Work out the finished part from the listing and answer in its coordinate system (mm). Round coordinates to 2 decimals unless told otherwise and drop trailing zeros. Loops run counter-clockwise (first coordinate to the right, second up) from the corner with the lowest first, then second, coordinate; pieces in that order, holes last. Notation, with made-up numbers: (-26, 33.25) -> (8, 33.25) arc R5 ccw to (8, 38.25) -> close; hole circle Ø4 at (-9.5, -2.75). An arc over 180 degrees is marked (long way). Write item = value, one per line. Start each with the question number.
```python
from build123d import *

# Parameters (mm, degrees)
BOSS_EXTRUDE1_DEPTH  = 3
M5_CLEARANCE_HOLE1_D = 5.5
M5_CLEARANCE_HOLE2_D = 5.5
M5_CLEARANCE_HOLE3_D = 5.5
FILLET2_R            = 2.5


with BuildPart() as part:
    # Sketch1 → Boss-Extrude1 (new body)
    with BuildSketch(Plane.XY):
        with BuildLine():
            Line((8.695255676, -3.826555727), (2.390511351, -18.153111454))
            ThreePointArc((2.390511351, -18.153111454), (-4.61754166, -26.412402673), (-15, -29.5))
            Line((-15, -29.5), (-51.88, -29.5))
            Line((-51.88, -29.5), (-51.88, -10.5))
            Line((-51.88, -10.5), (-15, -10.5))
            Line((-15, -10.5), (-8.695255676, 3.826555727))
            ThreePointArc((-8.695255676, 3.826555727), (3.826555727, 8.695255676), (8.695255676, -3.826555727))
        make_face()
    extrude(amount=BOSS_EXTRUDE1_DEPTH)

    # M5 Clearance Hole1 (through all)
    with Locations(Plane.XY.offset(3)):
        with Locations((-43.44, -20)):
            Hole(M5_CLEARANCE_HOLE1_D / 2)

    # M5 Clearance Hole2 (through all)
    with Locations(Plane.XY.offset(3)):
        with Locations((-23.44, -20)):
            Hole(M5_CLEARANCE_HOLE2_D / 2)

    # M5 Clearance Hole3 (through all)
    with Locations(Plane.XY.offset(3)):
        with Locations((0, 0)):
            Hole(M5_CLEARANCE_HOLE3_D / 2)

    # Fillet2
    fillet2_edges = [part.edges().sort_by_distance(p)[0] for p in [
        (-51.88, -29.5, 1.5),
        (-51.88, -10.5, 1.5),
        (-15, -10.5, 1.5),
    ]]
    fillet(fillet2_edges, radius=FILLET2_R)


solid = part.part
```
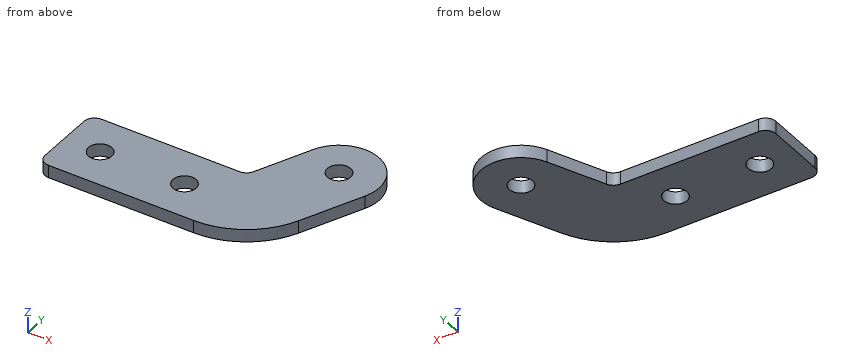
Item 1: Section A-A (x = -23.44) is taken. Determine the outline of the cut face in (y, z), then the cut area to 3 significant figures.
Item 2: Section B-B (z = 1.25) is taken. Determine the outline of the cut face in (x, y).
Item 3: Find the intervals of material crossed by line 1 along Y through (x, z) = (-23.44, 1.1); line 2 along X through (y, z) = (-17.5, 1.9); line 3 along X through (y, z) = (-22, 2.55), in increasing order. Write a range as [from, to].
Item 4: Flat-ended cylindrical pins translate along their axes: pin 1 (1.5 mm diameter, centred on y = 2.5, z = 1, fed in from +X); pin 2 (1.5 mm diameter, centred on x = -40, z = 1, fed in from +Y). Find the tip coordinate at first contact, or state that the pin passes through.
Item 5: Section C-C (y = -20) is taken. Determine the outline of the cut face in (x, z), then the cut area to 3 significant figures.
Item 6: Section D-D (y = 0) is taken. Determine the outline of the cut face in (x, z).
Worked answers:
q1.outline = (-29.5, 0) -> (-22.75, 0) -> (-22.75, 3) -> (-29.5, 3) -> close; (-17.25, 0) -> (-10.5, 0) -> (-10.5, 3) -> (-17.25, 3) -> close
q1.area = 40.5 mm2
q2.outline = (-51.88, -27) arc R2.5 ccw to (-49.38, -29.5) -> (-15, -29.5) arc R19 ccw to (2.39, -18.15) -> (8.7, -3.83) arc R9.5 ccw to (-8.7, 3.83) -> (-14.34, -9.01) arc R2.5 cw to (-16.63, -10.5) -> (-49.38, -10.5) arc R2.5 ccw to (-51.88, -13) -> close; hole circle Ø5.5 at (-43.44, -20); hole circle Ø5.5 at (-23.44, -20); hole circle Ø5.5 at (0, 0)
q3.line_1 = [-29.5, -22.75], [-17.25, -10.5]
q3.line_2 = [-51.88, -44.59], [-42.29, -24.59], [-22.29, 2.68]
q3.line_3 = [-51.88, -45.33], [-41.55, -25.33], [-21.55, 0.12]
q4.pin_1 = 9.34
q4.pin_2 = -10.5
q5.outline = (-51.88, 0) -> (-46.19, 0) -> (-46.19, 3) -> (-51.88, 3) -> close; (-40.69, 0) -> (-26.19, 0) -> (-26.19, 3) -> (-40.69, 3) -> close; (-20.69, 0) -> (1.45, 0) -> (1.45, 3) -> (-20.69, 3) -> close
q5.area = 127 mm2
q6.outline = (-10.38, 0) -> (-2.75, 0) -> (-2.75, 3) -> (-10.38, 3) -> close; (2.75, 0) -> (9.5, 0) -> (9.5, 3) -> (2.75, 3) -> close
